from build123d import *

# Parameters (mm, degrees)
F0_R     = 49.4974746831
F0_W     = 10
F0_H     = 4.9
F0_W_2   = 3
F0_H_2   = 10
F0_H_3   = 3.05
F1_DEPTH = 3


with BuildPart() as f1:
    # F0 (on Top) → F1 (new body)
    with BuildSketch(Plane.XY):
        Circle(F0_R)
        with Locations((-19.9997237325, -32.55)):
            Rectangle(F0_W, F0_H, mode=Mode.SUBTRACT)
        with Locations((-33.5, -20)):
            Rectangle(F0_W_2, F0_H_2, mode=Mode.SUBTRACT)
        with Locations((0.0002762675, -32.55)):
            Rectangle(F0_W, F0_H, mode=Mode.SUBTRACT)
        with Locations((20.0002762675, -32.55)):
            Rectangle(F0_W, F0_H, mode=Mode.SUBTRACT)
        with BuildLine():
            ThreePointArc((18.5589292605, 6.7548978307), (0, -19.75), (-18.5589292605, 6.7548978307))
            Line((-18.5589292605, 6.7548978307), (-12.9207735358, 4.7027769707))
            ThreePointArc((-12.9207735358, 4.7027769707), (0, -13.75), (12.9207735358, 4.7027769707))
            Line((12.9207735358, 4.7027769707), (18.5589292605, 6.7548978307))
        make_face(mode=Mode.SUBTRACT)
        with Locations((33.5, -20)):
            Rectangle(F0_W_2, F0_H_2, mode=Mode.SUBTRACT)
        with Locations((-33.5, 0)):
            Rectangle(F0_W_2, F0_H_2, mode=Mode.SUBTRACT)
        with Locations((-33.5, 20)):
            Rectangle(F0_W_2, F0_H_2, mode=Mode.SUBTRACT)
        with Locations((-20, 33.475)):
            Rectangle(F0_W, F0_H_3, mode=Mode.SUBTRACT)
        with BuildLine():
            ThreePointArc((-1.5, 2), (0, 2.5), (1.5, 2))
            Line((1.5, 2), (1.5, -2))
            ThreePointArc((1.5, -2), (0, -2.5), (-1.5, -2))
            Line((-1.5, -2), (-1.5, 2))
        make_face(mode=Mode.SUBTRACT)
        with Locations((33.5, 0)):
            Rectangle(F0_W_2, F0_H_2, mode=Mode.SUBTRACT)
        with Locations((33.5, 20)):
            Rectangle(F0_W_2, F0_H_2, mode=Mode.SUBTRACT)
        with Locations((0, 33.475)):
            Rectangle(F0_W, F0_H_3, mode=Mode.SUBTRACT)
        with Locations((20, 33.475)):
            Rectangle(F0_W, F0_H_3, mode=Mode.SUBTRACT)
    extrude(amount=F1_DEPTH)


solid = f1.part
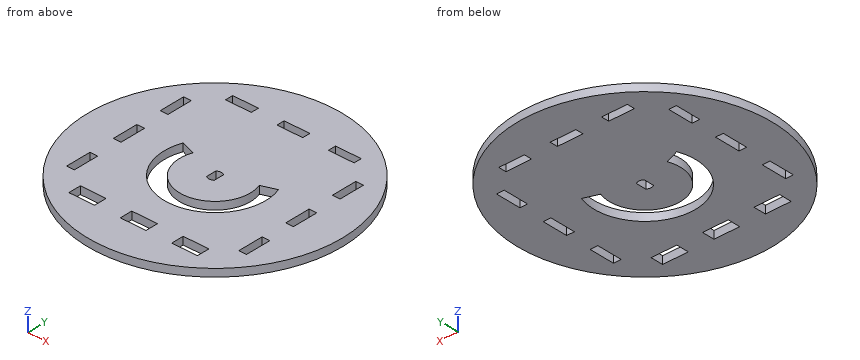
Geometry check sheet. Reference: the model listing, model coordinates, mm. Round coordinates to 2 decimals unless told otherwise and drop trailing zeros. Order: outer loops, then holes, each group sorted by start corner. A loop starts at its lowest first (then second) coordinate and runs counter-clockwise, first axis right, second up. Notation, with made-up numbers: (15.5, -33.75) - (74.5, -33.75) arc R16 cw to (74.5, -8.75) - close; hole circle Ø5 at (83, 51.5). An arc over 180 degrees is marked (long way). One line per question, with ' | ' between items. Start each with the question number.
(1) Depth check by flat-ended pin: pin 1 Ø1.5 at (x, z) = (-34, 1.5) entering from +Y; pin 2 Ø1 at (y, z) = (-31, 1.5) entering from +X; pin 3 Ø1.5 at (y, z) = (21.5, 1) entering from +X. Enter the tip coordinate at first touch or a pass-through.
(2) Thickness scan on L1, parallel to Y at x = -20, z = 2.7; L2, parallel to Y at x = 3, z = 2.85; L3, parallel to X at y = 20, z = 1.3. Record the ranges inside material, lowest first. Write a range as [from, to].
(3) Sectioned sample at A-A on x = 0. Record the cut outline in (y, z), and give its area (3 significant figures).
(4) Sectioned sample at B-B on y = 0. Record the cut outline in (x, z).
(5) Sectioned sample at D-D on z = 1.3. Count the separate pieces of the cut face and the enclosed holes in it, and give its area (3 significant figures).
(6) Sectioned sample at C-C on y = 18.5. Record the cut outline in (x, z), and give its area (3 significant figures).
Conclusion:
1) pin 1: stops at y = 36.67 | pin 2: stops at x = 38.98 | pin 3: stops at x = 44.94
2) L1: y = [-45.28, -35], [-30.1, 31.95], [35, 45.28] | L2: y = [-49.41, -35], [-30.1, -19.52], [-13.42, 31.95], [35, 49.41] | L3: x = [-45.28, -35], [-32, 32], [35, 45.28]
3) outline: (-49.5, 0) - (-35, 0) - (-35, 3) - (-49.5, 3) - close; (-30.1, 0) - (-19.75, 0) - (-19.75, 3) - (-30.1, 3) - close; (-13.75, 0) - (-2.5, 0) - (-2.5, 3) - (-13.75, 3) - close; (2.5, 0) - (31.95, 0) - (31.95, 3) - (2.5, 3) - close; (35, 0) - (49.5, 0) - (49.5, 3) - (35, 3) - close | area: 240 mm2
4) outline: (-49.5, 0) - (-35, 0) - (-35, 3) - (-49.5, 3) - close; (-32, 0) - (-19.75, 0) - (-19.75, 3) - (-32, 3) - close; (-13.75, 0) - (-1.5, 0) - (-1.5, 3) - (-13.75, 3) - close; (1.5, 0) - (13.75, 0) - (13.75, 3) - (1.5, 3) - close; (19.75, 0) - (32, 0) - (32, 3) - (19.75, 3) - close; (35, 0) - (49.5, 0) - (49.5, 3) - (35, 3) - close
5) separate pieces: 1 | enclosed holes: 14 | area: 6,880 mm2
6) outline: (-45.91, 0) - (-35, 0) - (-35, 3) - (-45.91, 3) - close; (-32, 0) - (32, 0) - (32, 3) - (-32, 3) - close; (35, 0) - (45.91, 0) - (45.91, 3) - (35, 3) - close | area: 257 mm2
